Here's how the part is built. I have some questions about the finished solid (model axes, mm). A direction names the side the tool comes from. Coordinates: 2 decimals unless noted, no trailing zeros. Write each loop counter-clockwise with the first axis right and the second up, starting at its lowest first coordinate (ties: lowest second). Pieces come first, ordered by that corner, then holes.
Item 1: For faces 4 (the face through (14.005, 0.493, -15.38)), 5 (the face through (0, 1, -48)), which set-ups out of +Z, -Z, +X, -X, +Y, -Y let a thin tool reach every point of the face, with its end or its side?
Item 2: We'd pull the mould along Z, two halves only. Please class faces 1 (the face through (-14.403, 0.493, -15.816)), 2 (the face through (14.734, 0.493, -13.21)), 3 (the face through (0, 0, -48)): +Z half, -Z half, draft (parallel to the pull), parting line (faces both ways), or undercut.
Item 3: If I drill on line 1 (X direction, y = 0.7, z = -47.5); line 2 (Z direction, x = -27, y = 0.2); line 3 (Z direction, x = 3.5, y = 0.45), over which ranges is the centre line in solid material (lowest first)?
Item 4: If we section it at C-C (z = -12.5): Please give me the cut outline in (x, y), then the cut area to 3 significant figures.
Item 5: If we section it at D-D (y = 0.65): Please give me the cut outline in (x, z), then the cut area to 3 significant figures.
Item 6: If we section it at B-B (x = 21): Please give me the cut outline in (y, z).
Item 7: If we section it at A-A (z = -53): Please give me the cut outline in (x, y).
Item 8: I'm going to push a flat-ended pin straight in: pin 1 Ø12 at (x, z) = (17.5, -47) entering from +Y. Where does the tip first touch, or does it pass through?
from build123d import *

# Parameters (mm, degrees)
BOSS_EXTRUDE2_DEPTH = 1


with BuildPart() as part:
    # Sketch1 → Boss-Extrude2 (new body)
    with BuildSketch(Plane(origin=(0, 0, 0), x_dir=(1, 0, 0), z_dir=(0, 1, 0))):
        with BuildLine():
            Line((0, -2.970477964), (29.886420182, 29.84931356))
            ThreePointArc((29.886420182, 29.84931356), (26.834835807, 57.297903562), (0, 50.768826482))
            ThreePointArc((0, 50.768826482), (-26.834835807, 57.297903562), (-29.886420182, 29.84931356))
            Line((-29.886420182, 29.84931356), (0, -2.970477964))
        make_face()
        with BuildLine():
            Line((0, 0), (28.407667395, 31.1958982))
            ThreePointArc((28.407667395, 31.1958982), (23.047800089, 57.163629593), (0, 44.054466297))
            ThreePointArc((0, 44.054466297), (-23.047800089, 57.163629593), (-28.407667395, 31.1958982))
            Line((-28.407667395, 31.1958982), (0, 0))
        make_face(mode=Mode.SUBTRACT)
    extrude(amount=BOSS_EXTRUDE2_DEPTH)


solid = part.part
Answer list:
1. face 4: +Y, -Y
1. face 5: +Z, -Z, +X, -X, +Y
2. face 1: undercut
2. face 2: +Z half
2. face 3: draft
3. line 1: x = -33.91 to -31.81, -0.77 to 0.77, 31.81 to 33.91
3. line 2: z = -57.18 to -54.64, -29.65 to -26.68
3. line 3: z = -55.45 to -52.48, -3.84 to -0.87
4. outline: (-14.09, 0) - (-11.38, 0) - (-11.38, 1) - (-14.09, 1) - close; (11.38, 0) - (14.09, 0) - (14.09, 1) - (11.38, 1) - close
4. area: 5.41 mm2
5. outline: (-29.89, -29.85) arc R18.39 ccw (long way) to (0, -50.77) arc R18.39 ccw (long way) to (29.89, -29.85) - (0, 2.97) - close; hole (-28.41, -31.2) arc R16.39 ccw (long way) to (0, -44.05) arc R16.39 ccw (long way) to (28.41, -31.2) - (0, 0) - close
5. area: 419 mm2
6. outline: (0, -60.01) - (1, -60.01) - (1, -57.93) - (0, -57.93) - close; (0, -23.06) - (1, -23.06) - (1, -20.09) - (0, -20.09) - close
7. outline: (-31.2, 0) - (-28.65, 0) - (-28.65, 1) - (-31.2, 1) - close; (-3.93, 0) - (-1.38, 0) - (-1.38, 1) - (-3.93, 1) - close; (1.38, 0) - (3.93, 0) - (3.93, 1) - (1.38, 1) - close; (28.65, 0) - (31.2, 0) - (31.2, 1) - (28.65, 1) - close
8. pin 1: passes through
